Input: part model. Units: mm. Frame: model coordinates. Give positions to 0.01 mm unless a question says otherwise; leave off trailing zeros. Loops run counter-clockwise (first coordinate to the right, second up) from the corner with the lowest first, then second, coordinate; pieces in that order, holes last. Notation, with made-up numbers: (-12.5, -10.5) -> (35.5, -10.5) arc R11 ccw to (35.5, 9.5) -> close; hole circle Ø7 at (41.25, 23.25). An arc over 180 degrees is marked (long way). Answer as a JSON object with one key per item and string values. Group by question number.
```python
from build123d import *

# Parameters (mm, degrees)
BOSS_EXTRU_1_DEPTH = 18
CONG_1_R           = 7


with BuildPart() as part:
    # Esquisse2 → Boss.-Extru.1 (new body)
    with BuildSketch(Plane.XY):
        with BuildLine():
            Line((-7.891319926, 50), (12.295896662, 50))
            Line((12.295896662, 50), (7.861291071, -0.687773849))
            ThreePointArc((7.861291071, -0.687773849), (-0.344214541, -7.883809138), (-7.891319926, 0))
            Line((-7.891319926, 0), (-7.891319926, 50))
        make_face()
    extrude(amount=BOSS_EXTRU_1_DEPTH)

    # Congé1
    cong_1_edges = [part.edges().sort_by_distance(p)[0] for p in [
        (-7.891319926, 50, 9),
        (12.295896662, 50, 9),
    ]]
    fillet(cong_1_edges, radius=CONG_1_R)


solid = part.part
```
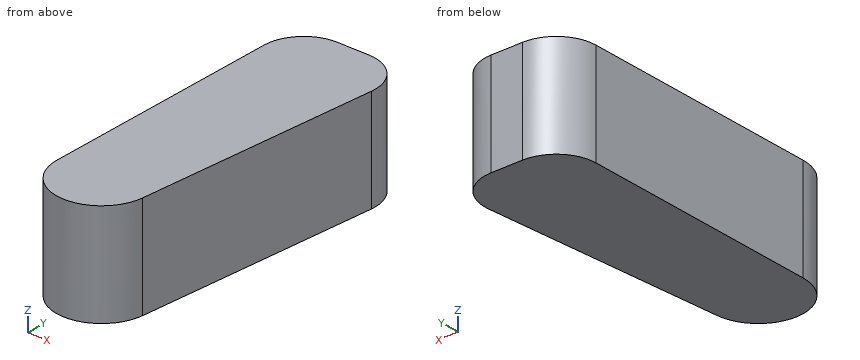
Q1. Section A-A on z = 10.75. Return the cut outline in (x, y).
Q2. Section C-C on y = 23. Return the cut outline in (x, z).
Q3. Section B-B on x = 9. Return the cut outline in (y, z).
Q4. Ray query, probe 1 along Y at (x, z) = (5.5, 12); probe 2 along X at (y, z) = (9, 2.5); probe 3 along Y at (x, z) = (6.5, 14). Return the intervals inside material, ascending.
Q5. Pin query (flat end, axial travel): pin 1 Ø1 at (x, y) = (9.5, 0.5) entering from -Z; pin 2 Ø1.5 at (x, z) = (-3, 12.5) entering from +Y. Return the tip coordinate at first contact, or that it passes through.
Numbers:
{
 "1": {"outline": "(-7.89, 0) arc R7.89 ccw to (7.86, -0.69) -> (11.63, 42.39) arc R7 ccw to (4.66, 50) -> (-0.89, 50) arc R7 ccw to (-7.89, 43) -> close"},
 "2": {"outline": "(-7.89, 0) -> (9.93, 0) -> (9.93, 18) -> (-7.89, 18) -> close"},
 "3": {"outline": "(12.33, 0) -> (48.49, 0) -> (48.49, 18) -> (12.33, 18) -> close"},
 "4": {"probe 1": "y = -5.66 to 49.95", "probe 2": "x = -7.89 to 8.71", "probe 3": "y = -4.47 to 49.75"},
 "5": {"pin 1": "passes through", "pin 2": "stops at y = 49.87"}
}
